```python
from build123d import *

# Parameters (mm, degrees)
SKETCH2_W           = 150
SKETCH2_H           = 50
BOSS_EXTRUDE1_DEPTH = 7.5
SKETCH3_R           = 1.475
CUT_EXTRUDE1_DEPTH  = 159.291661183
SKETCH4_R           = 1.3
CUT_EXTRUDE2_DEPTH  = 159.291661183
SKETCH6_W           = 140
SKETCH6_H           = 40
CUT_EXTRUDE3_DEPTH  = 2.5
SKETCH8_W           = 72
SKETCH8_H           = 24.3
CUT_EXTRUDE4_DEPTH  = 159.291661183
SKETCH9_W           = 12
SKETCH9_H           = 12
CUT_EXTRUDE5_DEPTH  = 159.291661183


with BuildPart() as part:
    # Sketch2 → Boss-Extrude1 (new body)
    with BuildSketch(Plane(origin=(0, 0, 0), x_dir=(1, 0, 0), z_dir=(0, 1, 0))):
        with Locations((75, 25)):
            Rectangle(SKETCH2_W, SKETCH2_H)
    extrude(amount=BOSS_EXTRUDE1_DEPTH)

    # Sketch3 → Cut-Extrude1 (cut, through all)
    with BuildSketch(Plane(origin=(0, 7.5, 0), x_dir=(1, 0, 0), z_dir=(0, 1, 0))):
        with Locations(Location((15, 40.216322293, 0), (0, 0, 270))):
            Circle(SKETCH3_R)
        with Locations(Location((89.9, 40.216322293, 0), (0, 0, 270))):
            Circle(SKETCH3_R)
        with Locations(Location((89.9, 9.783677707, 0), (0, 0, 270))):
            Circle(SKETCH3_R)
        with Locations(Location((15, 9.783677707, 0), (0, 0, 270))):
            Circle(SKETCH3_R)
    extrude(amount=-CUT_EXTRUDE1_DEPTH, mode=Mode.SUBTRACT)

    # Sketch4 → Cut-Extrude2 (cut, through all)
    with BuildSketch(Plane(origin=(0, 7.5, 0), x_dir=(1, 0, 0), z_dir=(0, 1, 0))):
        with Locations(Location((112.738384592, 17.7, 0), (0, 0, 270))):
            Circle(SKETCH4_R)
        with Locations(Location((126.238384592, 17.7, 0), (0, 0, 270))):
            Circle(SKETCH4_R)
    extrude(amount=-CUT_EXTRUDE2_DEPTH, mode=Mode.SUBTRACT)

    # Sketch6 → Cut-Extrude3 (cut)
    with BuildSketch(Plane.XZ):
        with Locations((75, -25)):
            Rectangle(SKETCH6_W, SKETCH6_H)
    extrude(amount=-CUT_EXTRUDE3_DEPTH, mode=Mode.SUBTRACT)

    # Sketch8 → Cut-Extrude4 (cut, through all)
    with BuildSketch(Plane(origin=(0, 7.5, 0), x_dir=(1, 0, 0), z_dir=(0, 1, 0))):
        with Locations((52.45, 24.55)):
            Rectangle(SKETCH8_W, SKETCH8_H)
    extrude(amount=-CUT_EXTRUDE4_DEPTH, mode=Mode.SUBTRACT)

    # Sketch9 → Cut-Extrude5 (cut, through all)
    with BuildSketch(Plane(origin=(0, 7.5, 0), x_dir=(1, 0, 0), z_dir=(0, 1, 0))):
        with Locations((117.438384592, 25.7)):
            Rectangle(SKETCH9_W, SKETCH9_H)
    extrude(amount=-CUT_EXTRUDE5_DEPTH, mode=Mode.SUBTRACT)


solid = part.part
```
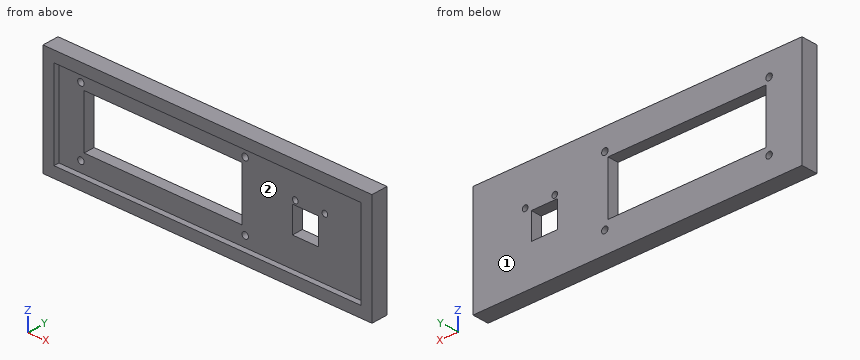
Could you check a few things on this model? Use its own coordinates, in mm. Face numbers are marked on the shaded views. Round coordinates to 2 decimals unless told otherwise and drop trailing zeros. Loops run counter-clockwise (first coordinate to the right, second up) from the corner with the lowest first, then second, coordinate; pieces in that order, holes last. Notation, with made-up numbers: (-35.75, 73.5) -> (21.25, 73.5) arc R13 ccw to (21.25, 81.5) -> close; hole circle Ø2 at (50, 28.5). An arc over 180 degrees is marked (long way). One line per question, with ' | ' between items.
(1) If we section it at B-B on x = 78.5: List the corners of the cut face in (y, z) for me, and give its area (4 significant figures).
Model answer:
outline: (0, -50) -> (7.5, -50) -> (7.5, -36.7) -> (2.5, -36.7) -> (2.5, -45) -> (0, -45) -> close; (0, -5) -> (2.5, -5) -> (2.5, -12.4) -> (7.5, -12.4) -> (7.5, 0) -> (0, 0) -> close | area: 153.5 mm^2
(2) If we section it at D-D on x = 109: List the corners of the cut face in (y, z) for me.
Model answer:
outline: (0, -50) -> (7.5, -50) -> (7.5, 0) -> (0, 0) -> (0, -5) -> (2.5, -5) -> (2.5, -45) -> (0, -45) -> close
(3) If we section it at A-A on z = -21: List the corners of the cut face in (x, y) for me, and give its area (3 significant figures).
Model answer:
outline: (0, 0) -> (5, 0) -> (5, 2.5) -> (16.45, 2.5) -> (16.45, 7.5) -> (0, 7.5) -> close; (88.45, 2.5) -> (111.44, 2.5) -> (111.44, 7.5) -> (88.45, 7.5) -> close; (123.44, 2.5) -> (145, 2.5) -> (145, 0) -> (150, 0) -> (150, 7.5) -> (123.44, 7.5) -> close | area: 355 mm^2
(4) If I drill on probe 1 along X at (y, z) = (3, -22); probe 2 along X at (y, z) = (1.25, -13.5); probe 3 along X at (y, z) = (6.5, -16), over which ranges is the centre line in solid material (lowest first)?
Model answer:
probe 1: x = 0 to 16.45, 88.45 to 111.44, 123.44 to 150 | probe 2: x = 0 to 5, 145 to 150 | probe 3: x = 0 to 16.45, 88.45 to 150
(5) If we section it at C-C on x = 15: List the corners of the cut face in (y, z) for me, and give its area (4 significant figures).
Model answer:
outline: (0, -50) -> (7.5, -50) -> (7.5, -41.69) -> (2.5, -41.69) -> (2.5, -45) -> (0, -45) -> close; (0, -5) -> (2.5, -5) -> (2.5, -8.31) -> (7.5, -8.31) -> (7.5, 0) -> (0, 0) -> close; (2.5, -38.74) -> (7.5, -38.74) -> (7.5, -11.26) -> (2.5, -11.26) -> close | area: 245.5 mm^2
(6) Thinking about a two-plate mould opening in X: for the marked faces 1 and 2, which applies, released by +X, released by -X, zero draft, split by the parting line, or undercut?
Model answer:
face 1: zero draft | face 2: undercut
(7) For pin 1 Ø1.5 at (x, y) = (35.5, 2) entering from +Z; pin 2 Ø2.5 at (x, z) = (15, -9.78) entering from +Y; pin 3 Ø4.5 at (x, z) = (89.9, -9.78) entering from -Y, each with a flat end and sliding along its axis, tell me the tip position at first contact or that it passes through.
Model answer:
pin 1: stops at z = 0 | pin 2: passes through | pin 3: stops at y = 2.5
